```python
from build123d import *

# Parameters (mm, degrees)
BOX058_W     = 10
BOX058_H     = 4
BOX058_DEPTH = 7.7
BOX057_W     = 43.18
BOX057_H     = 1.5
BOX057_DEPTH = 17.78
BOX069_W     = 5
BOX069_H     = 8.2
BOX069_DEPTH = 8


with BuildPart() as cube057:
    # Box058 → Box058 (new body)
    with BuildSketch(Plane(origin=(34, 18.5, 47), x_dir=(1, 0, 0), z_dir=(0, 0, 1))):
        with Locations((5, 2)):
            Rectangle(BOX058_W, BOX058_H)
    extrude(amount=BOX058_DEPTH)


with BuildPart() as fusion025:
    # Box057 → Box057 (new body)
    with BuildSketch(Plane(origin=(-1.5, 22.5, 42), x_dir=(1, 0, 0), z_dir=(0, 0, 1))):
        with Locations((21.59, 0.75)):
            Rectangle(BOX057_W, BOX057_H)
    extrude(amount=BOX057_DEPTH)

    # Fusion017: union Cube057
    add(cube057.part)


with BuildPart() as arduino:
    # Box069 → Box069 (new body)
    with BuildSketch(Plane(origin=(-1.5, 14.3, 47), x_dir=(1, 0, 0), z_dir=(0, 0, 1))):
        with Locations((2.5, 4.1)):
            Rectangle(BOX069_W, BOX069_H)
    extrude(amount=BOX069_DEPTH)

    # Fusion020: union Fusion025
    add(fusion025.part)


with BuildPart() as arduino_1:
    # Fusion020 placement: moved
    add(arduino.part.moved(Location((26, -10, -0.6))))


solid = arduino_1.part
```
Can you work these out from the model? Positions are in its coordinate system, mm. A direction names the side the tool comes from. Round coordinates to 2 decimals unless told otherwise and drop trailing zeros. Order: outer loops, then holes, each group sorted by start corner. A loop starts at its lowest first (then second) coordinate and runs counter-clockwise, first axis right, second up.
(1) If I drill on L1, parallel to X at y = 9, z = 52.75; L2, parallel to Y at x = 57, z = 53; L3, parallel to Z at x = 61, y = 11, over which ranges is the centre line in solid material (lowest first)?
Results are:
L1: x = 24.5 to 29.5, 60 to 70
L2: y = 12.5 to 14
L3: z = 46.4 to 54.1
(2) If we section it at A-A (y = 11): Please give me the cut outline in (x, z).
Results are:
outline: (24.5, 46.4) - (29.5, 46.4) - (29.5, 54.4) - (24.5, 54.4) - close; (60, 46.4) - (70, 46.4) - (70, 54.1) - (60, 54.1) - close
(3) On a 3-axis mill with a long thin cutter (end or side, diameter ignored), from which of +Z, -Z, +X, -X, +Y, -Y can I reach the whole of each face in a straight line? I mean faces 1 (the face through (29.5, 8, 50)), 2 (the face through (65, 8.5, 50)), 3 (the face through (65, 11, 46.4)), 4 (the face through (27, 8, 54.4)). Say none if no direction works.
Results are:
face 1: +Z, -Z, -Y
face 2: +Z, -Z, +X, -Y
face 3: -Z, +X, -X, -Y
face 4: +Z, +X, -X, -Y
(4) If we section it at D-D (y = 6): Please give me the cut outline in (x, z).
Results are:
outline: (24.5, 46.4) - (29.5, 46.4) - (29.5, 54.4) - (24.5, 54.4) - close
(5) I'm going to push flat-ended pins straight in: pin 1 (2 mm diameter, centred on x = 63.5, y = 10, fed in from +Z); pin 2 (2 mm diameter, centred on x = 64.5, y = 10, fed in from -Z); pin 3 (5.5 mm diameter, centred on x = 26, y = 6.5, fed in from +Z). Where does each tip first touch, or does it pass through?
Results are:
pin 1: stops at z = 54.1
pin 2: stops at z = 46.4
pin 3: stops at z = 54.4
(6) We'd pull the mould along X, two halves only. Please class faces 5 (the face through (27, 8, 46.4)), 6 (the face through (60, 10, 50)), 7 (the face through (70, 10, 50)): +X half, -X half, draft (parallel to the pull), parting line (faces both ways), or undercut.
Results are:
face 5: draft
face 6: undercut
face 7: +X half
(7) If we section it at B-B (x = 61): Please give me the cut outline in (y, z).
Results are:
outline: (8.5, 46.4) - (12.5, 46.4) - (12.5, 41.4) - (14, 41.4) - (14, 59.18) - (12.5, 59.18) - (12.5, 54.1) - (8.5, 54.1) - close
(8) If we section it at C-C (z = 53): Please give me the cut outline in (x, y), plus the area to 3 significant figures.
Results are:
outline: (24.5, 4.3) - (29.5, 4.3) - (29.5, 12.5) - (60, 12.5) - (60, 8.5) - (70, 8.5) - (70, 12.5) - (67.68, 12.5) - (67.68, 14) - (24.5, 14) - close
area: 146 mm2
